Here's the drawing with two shaded views (mm, measured from the low corner). I have some questions. Coordinates: 2 decimals unless noted, no trailing zeros. Write each loop counter-clockwise with the first axis right and the second up, starting at its lowest first coordinate (ties: lowest second). Pieces come first, ordered by that corner, then holes. Notation, with made-up numbers: (18, 24) -> (44, 24) arc R24 cw to (44, 42) -> close; hole circle Ø3 at (13.25, 10.25). An arc over 180 degrees is marked (long way). Use a Markdown table: item, result. Add a question column.
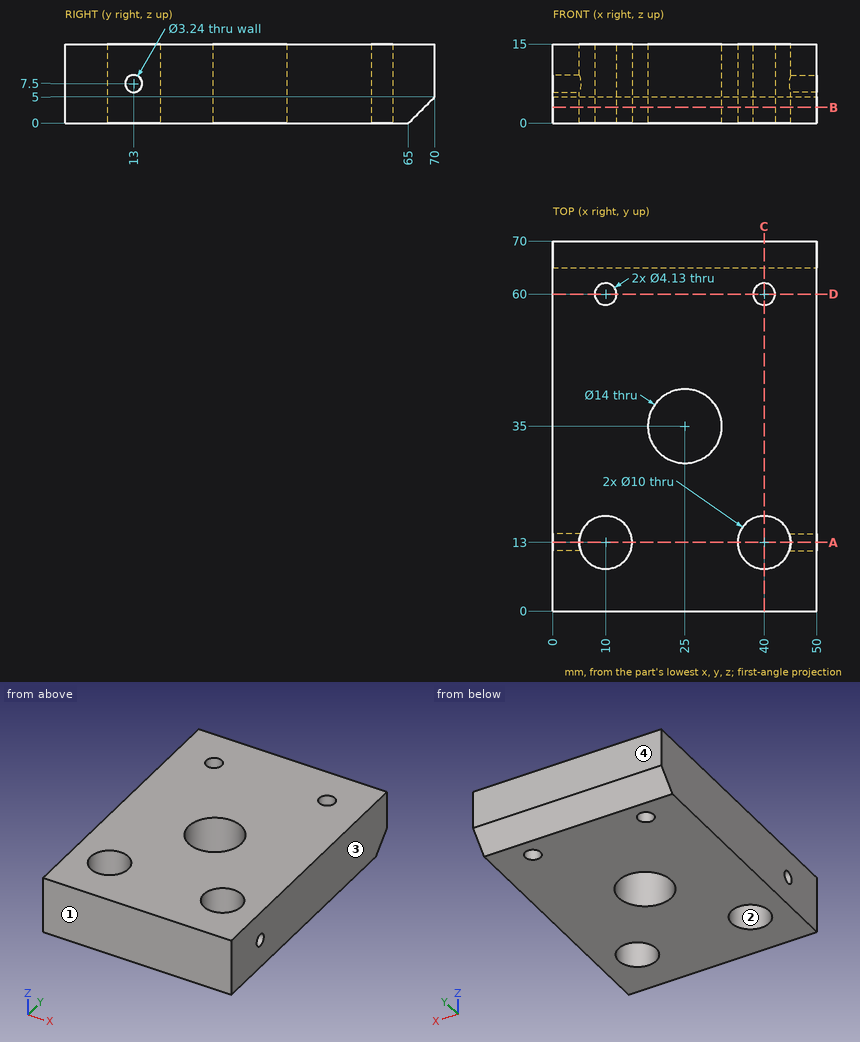
Q1. Suppose I cut it at A-A, the plane y = 13. Write out the boundary of the cut face in (x, z).
Q2. Suppose I cut it at B-B, the plane z = 3. Write out the boundary of the cut face in (x, y) (3 decimals), and give its area (3 significant figures).
Q3. Please list where these lines run through material, in increasing order: line 1 (Y direction, x = 40, z = 5.75) (3 decimals); line 2 (X direction, y = 10, z = 11); line 3 (Y direction, x = 25, z = 8.25).
Q4. Thinking about a two-plate mould opening in Y: for the marked faces 1, 2, 3 and 4, which applies, released by +Y, released by -Y, zero draft, split by the parting line, or undercut?
Q5. Will this pin go through, and if not, where does the flat tip stop? pin 1 (1.9 mm diameter, centred on y = 13, z = 7.5, fed in from -X).
Q6. Suppose I cut it at D-D, the plane y = 60. Write out the boundary of the cut face in (x, z) (3 decimals), and give its area (3 significant figures).
Q7. Suppose I cut it at C-C, the plane x = 40. Write out the boundary of the cut face in (y, z) (3 decimals).
Answer key:
| question | item | result |
|---|---|---|
| 1 | outline | (0, 0) -> (5, 0) -> (5, 5.88) -> (0, 5.88) -> close; (0, 9.12) -> (5, 9.12) -> (5, 15) -> (0, 15) -> close; (15, 0) -> (35, 0) -> (35, 15) -> (15, 15) -> close; (45, 0) -> (50, 0) -> (50, 5.88) -> (45, 5.88) -> close; (45, 9.12) -> (50, 9.12) -> (50, 15) -> (45, 15) -> close |
| 2 | outline | (0, 0) -> (50, 0) -> (50, 68) -> (0, 68) -> close; hole circle Ø10 at (10, 13); hole circle Ø4.13 at (10, 60); hole circle Ø14 at (25, 35); hole circle Ø10 at (40, 13); hole circle Ø4.13 at (40, 60) |
| 2 | area | 3,060 mm^2 |
| 3 | line 1 | y = 0 to 8, 18 to 57.935, 62.065 to 70 |
| 3 | line 2 | x = 0 to 6, 14 to 36, 44 to 50 |
| 3 | line 3 | y = 0 to 28, 42 to 70 |
| 4 | face 1 | released by -Y |
| 4 | face 2 | undercut |
| 4 | face 3 | zero draft |
| 4 | face 4 | released by +Y |
| 5 | pin 1 | stops at x = 14.91 |
| 6 | outline | (0, 0) -> (7.935, 0) -> (7.935, 15) -> (0, 15) -> close; (12.065, 0) -> (37.935, 0) -> (37.935, 15) -> (12.065, 15) -> close; (42.065, 0) -> (50, 0) -> (50, 15) -> (42.065, 15) -> close |
| 6 | area | 626 mm^2 |
| 7 | outline | (0, 0) -> (8, 0) -> (8, 15) -> (0, 15) -> close; (18, 0) -> (57.935, 0) -> (57.935, 15) -> (18, 15) -> close; (62.065, 0) -> (65, 0) -> (70, 5) -> (70, 15) -> (62.065, 15) -> close |
